Work out the finished part from the listing and answer in its coordinate system (mm). Round coordinates to 2 decimals unless told otherwise and drop trailing zeros. Order: outer loops, then holes, each group sorted by start corner. A loop starts at its lowest first (then second) coordinate and runs counter-clockwise, first axis right, second up. Notation, with made-up numbers: (69.5, -23.5) - (128.5, -23.5) arc R3 ccw to (128.5, -18.5) - close; hole circle Ø6 at (-23.5, 12.25). An arc over 180 degrees is marked (long way). Use one line per item in the form item = value. Start each with the question number.
Q1. The part is cut by section A-A on z = 0.2. Determine the outline of the cut face in (x, y).
Q2. The part is cut by section B-B on x = -43. Determine the outline of the cut face in (y, z).
Q3. Find the intervals of material crossed by line 1 (Y direction, x = -51.5, z = 0.85); line 2 (X direction, y = 59, z = 0.25); line 3 (Y direction, x = 28, z = 0.7), in increasing order. Write a range as [from, to].
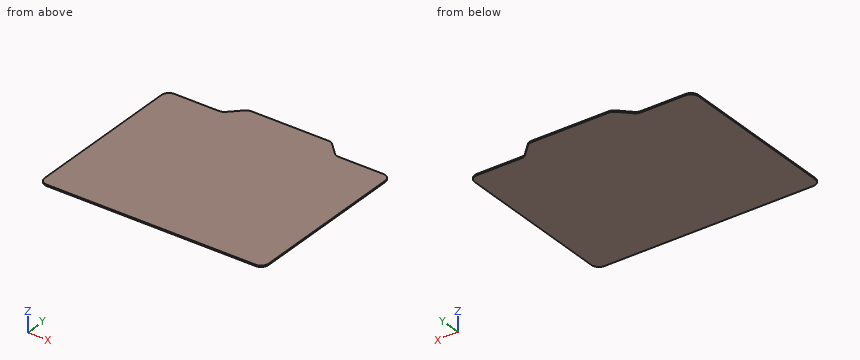
from build123d import *

# Parameters (mm, degrees)
F1_DEPTH = 0.9
F2_R     = 5


# Not quite as in the source:
# - a feature names something its author has since deleted; it is built from what else it names


with BuildPart() as f1:
    # F0 (on Top) → F1 (new body)
    with BuildSketch(Plane.XY):
        Polygon((-74, -59.5467374876), (74, -59.5467374876), (74, 55.4532625124), (37.5, 55.4532625124), (27.5, 65.4532625124), (-27.5, 65.4532625124), (-37.5, 55.4532625124), (-74, 55.4532625124), align=None)
    extrude(amount=F1_DEPTH)

    # F2
    f2_edges = [f1.edges().sort_by_distance(p)[0] for p in [
        (37.5, 55.453263, 0.45),
        (27.5, 65.453263, 0.45),
        (-37.5, 55.453263, 0.45),
        (-27.5, 65.453263, 0.45),
        (-74, 55.453263, 0.45),
        (-74, -59.546737, 0.45),
        (74, -59.546737, 0.45),
        (74, 55.453263, 0.45),
    ]]
    fillet(f2_edges, radius=F2_R)


solid = f1.part
Found:
q1.outline = (-74, -54.55) arc R5 ccw to (-69, -59.55) - (69, -59.55) arc R5 ccw to (74, -54.55) - (74, 50.45) arc R5 ccw to (69, 55.45) - (39.57, 55.45) arc R5 cw to (36.04, 56.92) - (28.96, 63.99) arc R5 ccw to (25.43, 65.45) - (-25.43, 65.45) arc R5 ccw to (-28.96, 63.99) - (-36.04, 56.92) arc R5 cw to (-39.57, 55.45) - (-69, 55.45) arc R5 ccw to (-74, 50.45) - close
q2.outline = (-59.55, 0) - (55.45, 0) - (55.45, 0.9) - (-59.55, 0.9) - close
q3.line_1 = [-59.55, 55.45]
q3.line_2 = [-33.95, 33.95]
q3.line_3 = [-59.55, 64.74]
